```python
from build123d import *

# Parameters (mm, degrees)
F1_DEPTH = 2.54
F3_DEPTH = 2.54
F5_DEPTH = 2.54
F7_DEPTH = 2.54
F9_DEPTH = 2.54


with BuildPart() as f1:
    # F0 (on Front) → F1 (new body)
    with BuildSketch(Plane.XZ):
        Polygon((0, 12.7), (0, 0), (17.78, 0), (17.78, 5.08), (5.08, 5.08), (5.08, 12.7), align=None)
    extrude(amount=F1_DEPTH)



with BuildPart() as f3:
    # F2 (on face) → F3 (new body)
    with BuildSketch(Plane(origin=(0, 5.08, 0), x_dir=(-1, 0, 0), z_dir=(0, 1, 0))):
        Polygon((-17.78, 0), (0, 0), (0, 10.16), (-5.08, 10.16), (-5.08, 5.08), (-17.78, 5.08), align=None)
    extrude(amount=F3_DEPTH)

    # F4 (on face) → F5 (join)
    with BuildSketch(Plane(origin=(0, 2.54, 0), x_dir=(-1, 0, 0), z_dir=(0, 1, 0))):
        Polygon((0, 0), (0, 10.16), (-5.08, 10.16), (-5.08, 5.08), (-10.16, 5.08), (-10.16, 0), align=None)
    extrude(amount=F5_DEPTH)


with BuildPart() as f1_1:
    add(f1.part)

    add(f3.part)  # F7 merges F3
    # F6 (on face) → F7 (join)
    with BuildSketch(Plane(origin=(0, 0, 0), x_dir=(-1, 0, 0), z_dir=(0, 1, 0))):
        Polygon((-17.78, 0), (0, 0), (0, 10.16), (-5.08, 10.16), (-5.08, 5.08), (-17.78, 5.08), align=None)
    extrude(amount=F7_DEPTH)

    # F8 (on face) → F9 (join)
    with BuildSketch(Plane(origin=(0, 7.62, 0), x_dir=(-1, 0, 0), z_dir=(0, 1, 0))):
        Polygon((-17.78, 0), (0, 0), (0, 12.7), (-5.08, 12.7), (-5.08, 5.08), (-17.78, 5.08), align=None)
    extrude(amount=F9_DEPTH)


solid = f1_1.part
```
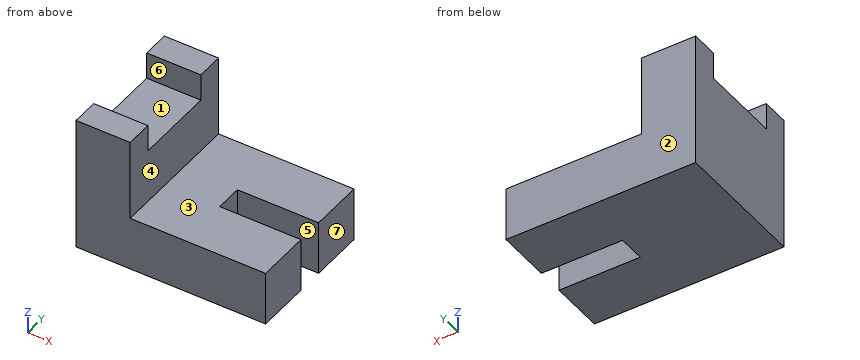
Can you work these out from the model? Positions are in its coordinate system, mm. Face numbers are marked on the shaded views. A direction names the side the tool comes from. Round coordinates to 2 decimals unless told otherwise and drop trailing zeros. Loops run counter-clockwise (first coordinate to the right, second up) from the corner with the lowest first, then second, coordinate; pieces in that order, holes last. Notation, with made-up numbers: M 29.25,58 L 79.25,58 A33 ccw 79.25,89 Z; hole C -36.5,84 d5. An arc over 180 degrees is marked long. Answer as a JSON object with one key per item and string values. Group by question number.
Q1. On a 3-axis mill with a long thin cutter (end or side, diameter ignored), from which of +Z, -Z, +X, -X, +Y, -Y can I reach the whole of each face in a straight line? I mean the marked faces 4, 5, 6 and 7. Say none if no direction works.
Q2. Will these pins go through, and if not, where does the flat tip stop? pin 1 (2.5 mm diameter, centred on x = 4, y = 4, fed in from +Z); pin 2 (6.5 mm diameter, centred on x = 11.5, y = 6, fed in from +Z).
Q3. Please list where these lines run through material, in increasing order: L1, parallel to Y at x = 11, z = 2; L2, parallel to X at y = 2.5, z = 6.
Q4. Imagine slicing it at A-A, the plane x = 13.75. Please give me the cut outline in (y, z).
Q5. Imagine slicing it at B-B, the plane z = 11.25. Please give me the cut outline in (x, y), then the cut area to 3 significant figures.
Q6. We'd pull the mould along Y, two halves only. Please class the marked faces 1, 2 and 3: +Y half, -Y half, draft (parallel to the pull), parting line (faces both ways), or undercut.
Q7. Imagine slicing it at C-C, the plane z = 3. Please give me the cut outline in (x, y).
Q8. Imagine slicing it at D-D, the plane y = 8.25. Please give me the cut outline in (x, z).
Findings:
{
 "1": {"face 4": "+Z, +X, +Y, -Y", "face 5": "+Z, -Z, +X", "face 6": "+Z, +X, -X", "face 7": "+Z, -Z, +X, +Y, -Y"},
 "2": {"pin 1": "stops at z = 10.16", "pin 2": "stops at z = 5.08"},
 "3": {"L1": "y = -2.54 to 2.54, 5.08 to 10.16", "L2": "x = 0 to 5.08"},
 "4": {"outline": "M -2.54,0 L 2.54,0 L 2.54,5.08 L -2.54,5.08 Z; M 5.08,0 L 10.16,0 L 10.16,5.08 L 5.08,5.08 Z"},
 "5": {"outline": "M 0,-2.54 L 5.08,-2.54 L 5.08,0 L 0,0 Z; M 0,7.62 L 5.08,7.62 L 5.08,10.16 L 0,10.16 Z", "area": "25.8 mm2"},
 "6": {"face 1": "undercut", "face 2": "+Y half", "face 3": "draft"},
 "7": {"outline": "M 0,-2.54 L 17.78,-2.54 L 17.78,2.54 L 10.16,2.54 L 10.16,5.08 L 17.78,5.08 L 17.78,10.16 L 0,10.16 Z"},
 "8": {"outline": "M 0,0 L 17.78,0 L 17.78,5.08 L 5.08,5.08 L 5.08,12.7 L 0,12.7 Z"}
}
